Read the model definition and answer for the solid it produces. Units are mm, in the model's axes. Give positions to 0.01 mm unless a question says otherwise; leave off trailing zeros. Write each loop counter-clockwise with the first axis right and the second up, starting at its lowest first coordinate (ties: lowest second). Pieces come first, ordered by that corner, then holes. Notation, with made-up numbers: (60, -21) -> (71, -21) arc R13 cw to (71, -12) -> close; hole circle Ø6 at (34.5, -4.5). An arc over 180 degrees is marked (long way). Put each result on its own line as item: value. Start each with the question number.
from build123d import *

# Parameters (mm, degrees)
SKETCH1_R      = 5.55625
EXTRUDE1_DEPTH = 3.175


with BuildPart() as part:
    # Sketch1 → Extrude1 (new body)
    with BuildSketch(Plane.XY):
        with BuildLine():
            Line((90.184030844, 0), (152.625697511, 0))
            ThreePointArc((152.625697511, 0), (155.107278383, 1.998376171), (153.684030844, 4.849010731))
            Line((153.684030844, 4.849010731), (90.184030844, 33.954188012))
            Line((90.184030844, 33.954188012), (90.184030844, 0))
        make_face()
        with Locations((120.875697511, 7.62)):
            Circle(SKETCH1_R, mode=Mode.SUBTRACT)
        with Locations((101.825697511, 7.62)):
            Circle(SKETCH1_R, mode=Mode.SUBTRACT)
    extrude(amount=EXTRUDE1_DEPTH)


solid = part.part
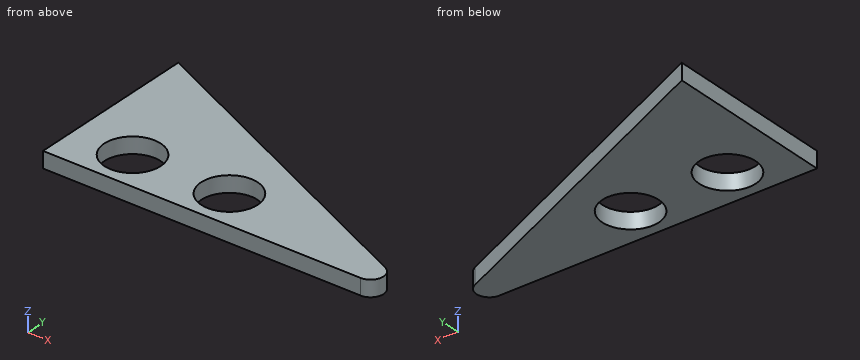
1) A cutting plane is placed at A-A on y = 11. Give the vertices of the cut face in (x, z) (3 decimals), and give its area (3 significant figures).
2) A cutting plane is placed at B-B on x = 121. Give the vertices of the cut face in (y, z) (3 decimals).
3) Straight lines are drawn through the part: line 1 (X direction, y = 8, z = 1.85); line 2 (Y direction, x = 101, z = 2.85); line 3 (Y direction, x = 98, z = 2.5). For each, find the intervals that lie inside material, in ascending order. Write a range as [from, to].
4) A cutting plane is placed at D-D on x = 98. Give the vertices of the cut face in (y, z) (3 decimals).
5) A cutting plane is placed at C-C on z = 1.2. Give the vertices of the cut face in (x, y), and give its area (3 significant figures).
6) Each of these flat-tipped pins is pushed along its axis until it touches: pin 1 Ø1.5 at (y, z) = (15.5, 0.5) entering from +X; pin 2 Ø1.5 at (y, z) = (27, 2) entering from +X; pin 3 Ø8 at (x, y) = (122.5, 26.5) entering from -Z. Where does it stop, or does it pass through?
Results found:
1. outline: (90.184, 0) -> (97.416, 0) -> (97.416, 3.175) -> (90.184, 3.175) -> close; (106.236, 0) -> (116.466, 0) -> (116.466, 3.175) -> (106.236, 3.175) -> close; (125.286, 0) -> (140.264, 0) -> (140.264, 3.175) -> (125.286, 3.175) -> close
1. area: 103 mm²
2. outline: (0, 0) -> (2.065, 0) -> (2.065, 3.175) -> (0, 3.175) -> close; (13.175, 0) -> (19.83, 0) -> (19.83, 3.175) -> (13.175, 3.175) -> close
3. line 1: x = [90.18, 96.28], [107.37, 115.33], [126.42, 146.81]
3. line 2: y = [0, 2.13], [13.11, 29]
3. line 3: y = [0, 3.59], [11.65, 30.37]
4. outline: (0, 0) -> (3.591, 0) -> (3.591, 3.175) -> (0, 3.175) -> close; (11.649, 0) -> (30.372, 0) -> (30.372, 3.175) -> (11.649, 3.175) -> close
5. outline: (90.18, 0) -> (152.63, 0) arc R2.54 ccw to (153.68, 4.85) -> (90.18, 33.95) -> close; hole circle Ø11.11 at (101.83, 7.62); hole circle Ø11.11 at (120.88, 7.62)
5. area: 1,040 mm²
6. pin 1: stops at x = 132.08
6. pin 2: stops at x = 106.99
6. pin 3: passes through
